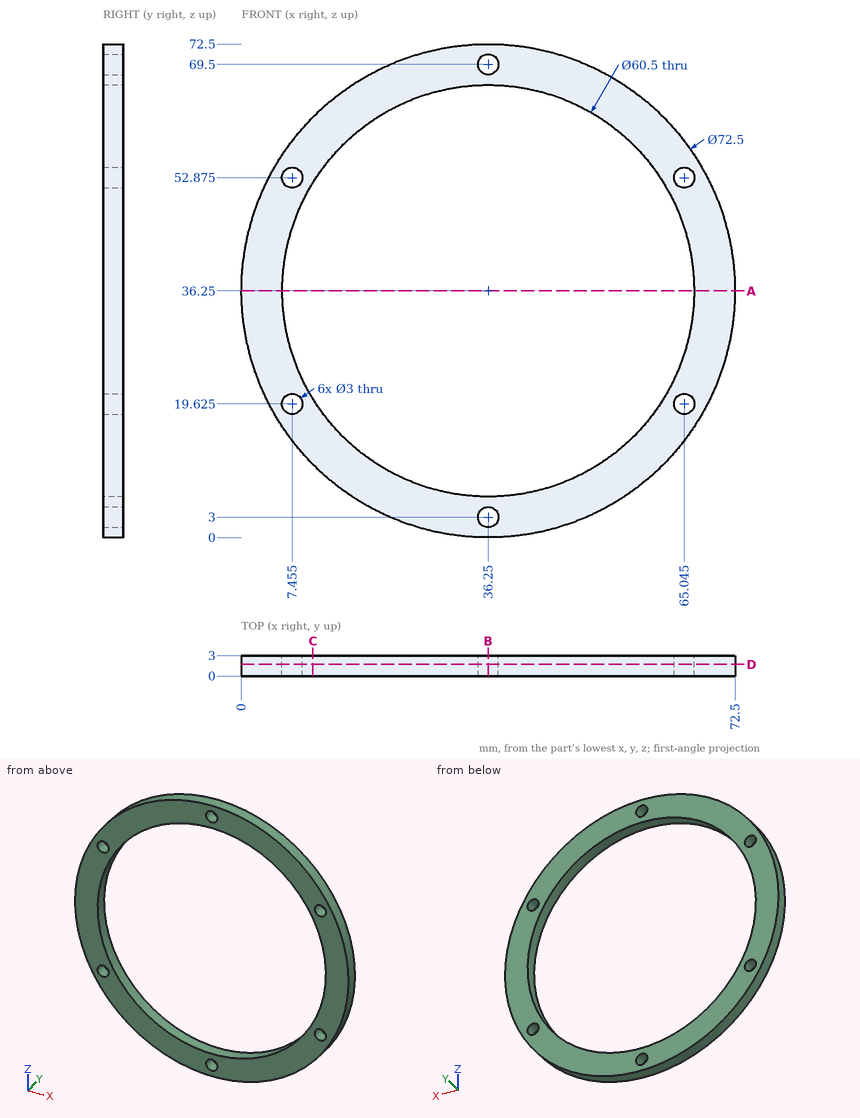
Can you work these out from the drawing? Everything is in mm from the part's minimum corner. Coordinates: 2 decimals unless noted, no trailing zeros. Loops run counter-clockwise (first coordinate to the right, second up) from the corner with the lowest first, then second, coordinate; pieces in that order, holes last. Notation, with made-up numbers: (64, 60.25) - (87, 60.25) arc R33 ccw to (87, 91.25) - close; hole circle Ø7 at (5, 25). An arc over 180 degrees is marked (long way). Use a Markdown table: item, result.
Item 1: I want a section at C-C on x = 10.5. Please give me the cut outline in (y, z) (1 decimal).
Numbers:
| item | result |
|---|---|
| outline | (0, 10.7) - (3, 10.7) - (3, 20.4) - (0, 20.4) - close; (0, 52.1) - (3, 52.1) - (3, 61.8) - (0, 61.8) - close |
Item 2: I want a section at B-B on x = 36.25. Please give me the cut outline in (y, z).
Numbers:
| item | result |
|---|---|
| outline | (0, 0) - (3, 0) - (3, 1.5) - (0, 1.5) - close; (0, 4.5) - (3, 4.5) - (3, 6) - (0, 6) - close; (0, 66.5) - (3, 66.5) - (3, 68) - (0, 68) - close; (0, 71) - (3, 71) - (3, 72.5) - (0, 72.5) - close |
Item 3: I want a section at D-D on y = 1.7. Give the number of separate pieces and of enclosed holes in the cut face, and give its area (3 significant figures).
Numbers:
| item | result |
|---|---|
| separate pieces | 1 |
| enclosed holes | 7 |
| area | 1,210 mm2 |
Item 4: I want a section at A-A on z = 36.25. Please give me the cut outline in (x, y).
Numbers:
| item | result |
|---|---|
| outline | (0, 0) - (6, 0) - (6, 3) - (0, 3) - close; (66.5, 0) - (72.5, 0) - (72.5, 3) - (66.5, 3) - close |
Item 5: Will these pins go through, and if not, where does the flat tip stop? pin 1 (4 mm diameter, centred on x = 40.5, z = 8, fed in from -Y); pin 2 (1.5 mm diameter, centred on x = 28.5, y = 1, fed in from +Z); pin 3 (1.5 mm diameter, centred on x = 20, y = 1, fed in from -Z).
Numbers:
| item | result |
|---|---|
| pin 1 | stops at y = 0 |
| pin 2 | stops at z = 71.82 |
| pin 3 | stops at z = 3.48 |
Item 6: If I drill on probe 1 along X at (y, z) = (1.05, 54) (1 decimal); probe 2 along X at (y, z) = (1.1, 53); probe 3 along X at (y, z) = (1.95, 36.25), over which ranges is the centre line in solid material (lowest first)? Write a range as from..to.
Numbers:
| item | result |
|---|---|
| probe 1 | x = 4.6..6.5, 8.4..11.8, 60.7..64.1, 66..67.9 |
| probe 2 | x = 4.1..5.96, 8.95..11.06, 61.44..63.55, 66.54..68.4 |
| probe 3 | x = 0..6, 66.5..72.5 |
